Autodesk Inventor part; units mm, degrees
ref_plane "YZ Plane" through (0, 0, 0) normal (1, 0, 0) x (0, 1, 0)
ref_plane "XZ Plane" through (0, 0, 0) normal (0, 1, 0) x (-1, 0, 0)
ref_plane "XY Plane" through (0, 0, 0) normal (0, 0, 1) x (1, 0, 0)
sketch "Sketch1" plane through (0, 0, 0) normal (0, 1, 0) x (-1, 0, 0)
  line L0 (4.75, 4) -> (-4.75, 4)
  line L1 (-4.75, 4) -> (-4.75, -4)
  line L2 (-4.75, -4) -> (4.75, -4)
  line L3 (4.75, -4) -> (4.75, 4)
  line L4 (4.75, 4) -> (-4.75, -4) construction
  line L5 (-4.75, 4) -> (4.75, -4) construction
  point P0 (0, 0)
  dimension "d0" = 9.5
  dimension "d1" = 8
extrude "Extrusion1" add sketch "Sketch1" along normal blind 8
sketch "Sketch2" plane through (0, 8, 0) normal (0, 1, 0) x (1, 0, 0)
  circle A0 centre (-0.45, 0) radius 2
  line L0 (-4.75, 4) -> (-4.75, -4)
  line L1 (4.75, 4) -> (-4.75, 4)
  point P0 (0, 0)
  dimension "d4" = 4
  dimension "d5" = 4.3
  dimension "d6" = 4
extrude "Extrusion2" add sketch "Sketch2" along normal blind 3.2
sketch "Sketch3" plane through (-0.45, 11.2, 0) normal (0, 1, 0) x (1, 0, 0)
  point P0 (0.45, 0)
  point P1 (0, 0)
hole "Hole1" at (-0.45, 11.2, 0) direction (0, -1, 0) diameter 2.5 depth 8
sketch "Sketch4" plane through (0, 0, 0) normal (0, -1, 0) x (1, 0, 0)
  line L0 (-3.65, -1) -> (-3.85, -1)
  line L1 (-3.85, -1) -> (-3.85, 1)
  line L2 (-3.85, 1) -> (-3.65, 1)
  line L3 (-3.65, 1) -> (-3.65, -1)
  line L4 (-3.65, -1) -> (-3.85, 1) construction
  line L5 (-3.85, -1) -> (-3.65, 1) construction
  line L6 (3.65, -1) -> (3.85, -1)
  line L7 (3.85, -1) -> (3.85, 1)
  line L8 (3.85, 1) -> (3.65, 1)
  line L9 (3.65, 1) -> (3.65, -1)
  line L10 (3.65, -1) -> (3.85, 1) construction
  line L11 (3.85, -1) -> (3.65, 1) construction
  line L12 (4.75, 4) -> (4.75, -4)
  line L13 (-4.75, 4) -> (4.75, 4)
  point P0 (0, 0)
  point P1 (-3.75, 0)
  point P2 (3.75, 0)
  point P3 (3.65, 0)
  dimension "d16" = 0.2
  dimension "d17" = 2
  dimension "d18" = 0.2
  dimension "d19" = 2
  dimension "d20" = 7.5
  dimension "d21" = 1
  dimension "d22" = 4
extrude "Extrusion3" add sketch "Sketch4" along normal blind 5
fillet "Fillet1" radius 1 4 edges at (3.75, -5, -1) (3.75, -5, 1) (-3.75, -5, 1) (-3.75, -5, -1)
sketch "Sketch5" plane through (3.85, 0, 1) normal (1, 0, 0) x (0, 0, -1)
  line L0 (1, -2) -> (1, -4) construction
  line L1 (1.5, -2) -> (1.5, -4)
  line L2 (0.5, -4) -> (0.5, -2)
  arc A0 (1.5, -2) -> (0.5, -2) centre (1, -2) ccw
  arc A1 (0.5, -4) -> (1.5, -4) centre (1, -4) ccw
  line L3 (0, 0) -> (0, -4)
  arc A2 (0, -4) -> (2, -4) centre (1, -4) ccw
  point P0 (1, 0)
  point P1 (1, -3)
  dimension "d26" = 1
  dimension "d27" = 1
  dimension "d28" = 0.5
  dimension "d29" = 0.5
extrude "Extrusion4" cut sketch "Sketch5" against normal through all
sketch "Sketch6" plane through (-4.75, 0, -4) normal (-1, 0, 0) x (0, 0, 1)
  line L0 (3, 7.6) -> (5, 7.6)
  line L1 (5, 7.6) -> (5, 7.4)
  line L2 (5, 7.4) -> (3, 7.4)
  line L3 (3, 7.4) -> (3, 7.6)
  line L4 (3, 7.6) -> (5, 7.4) construction
  line L5 (5, 7.6) -> (3, 7.4) construction
  line L6 (0, 0) -> (0, 8)
  line L7 (0, 8) -> (8, 8)
  point P0 (4, 0)
  point P1 (4, 7.5)
  dimension "d32" = 2
  dimension "d33" = 0.2
  dimension "d34" = 4
  dimension "d35" = 0.5
extrude "Extrusion5" add sketch "Sketch6" along normal blind 5.7
fillet "Fillet2" radius 1 2 edges at (-10.45, 7.5, 1) (-10.45, 7.5, -1)
sketch "Sketch7" plane through (-4.75, 7.6, 1) normal (0, 1, 0) x (1, 0, 0)
  line L0 (-4.7, 1) -> (-3.7, 1) construction
  line L1 (-4.7, 0.5) -> (-3.7, 0.5)
  line L2 (-3.7, 1.5) -> (-4.7, 1.5)
  arc A0 (-4.7, 1.5) -> (-4.7, 0.5) centre (-4.7, 1) ccw
  arc A1 (-3.7, 0.5) -> (-3.7, 1.5) centre (-3.7, 1) ccw
  line L3 (0, 2) -> (-4.7, 2)
  arc A2 (-4.7, 2) -> (-4.7, 0) centre (-4.7, 1) ccw
  point P0 (4.75, 1)
  point P1 (-4.2, 1)
  dimension "d39" = 0.5
  dimension "d40" = 1
  dimension "d41" = 0.5
  dimension "d42" = 0.5
extrude "Extrusion6" cut sketch "Sketch7" against normal through all
properties part number "2.5mm jack"
Part model, mm, in its own coordinate system. A direction names the side the tool comes from. Round coordinates to 2 decimals unless told otherwise and drop trailing zeros. Write each loop counter-clockwise with the first axis right and the second up, starting at its lowest first coordinate (ties: lowest second). Pieces come first, ordered by that corner, then holes. Notation, with made-up numbers: (-34, -28) -> (25, -28) arc R22 ccw to (25, 8) -> close; hole circle Ø3 at (52.25, -12.75). An arc over 180 degrees is marked (long way). Return JSON: item names as keys, results as strings. Group by question number.
Q1. Which spindle directions (+Z, -Z, +X, -X, +Y, -Y) get a long thin tool onto all of the face, cutting with end or side? Do faces 1 (the flat face through (3.85, -1.9, -0.7)), 2 (the cylindrical face through (0.77, 7.14, -0.27)), 3 (the flat face through (3.65, -1.9, 0.7)). Say none if no direction does.
Q2. Saw through at D-D on z = 2.5. Write the cut outline in (x, y), plus the area to 3 significant figures.
Q3. Probe L1, parallel to X at y = 9.25, z = 0; L2, parallel to X at y = 5, z = 0; L3, parallel to Z at x = -0.45, y = 9. List the from-to ranges inside material, lowest first. Write a range as [from, to].
Q4. Saw through at A-A on x = -8.25. Write the cut outline in (y, z).
Q5. Pin check, flat tips, straight feed: pin 1 (2 mm diameter, centred on y = -2.5, z = -0.5, fed in from -X); pin 2 (4 mm diameter, centred on y = 2.5, z = 0.5, fed in from -X); pin 3 (0.6 mm diameter, centred on y = -3, z = 0, fed in from +X) (3 decimals). Stop position of each tip, or through.
Q6. Saw through at B-B on y = 5.75. Write the cut outline in (x, z).
Q7. Mould opens along X. For faces 4 (the flat face through (-3.85, -1.9, -0.7)), 5 (the cylindrical face through (-0.884, 9.578, -1.952)), 6 (the flat face through (0, 3.2, 0)) say: pulls with the +X half, pulls with the -X half, needs draft (parallel to the pull), parting line crosses it, or undercut.
Q8. Saw through at C-C on x = -0.45. Write the cut outline in (y, z).
Answer:
{
 "1": {"face 1": "+Z, -Z, +X, -Y", "face 2": "+Y", "face 3": "+Z, -Z, -Y"},
 "2": {"outline": "(-4.75, 0) -> (4.75, 0) -> (4.75, 8) -> (-4.75, 8) -> close", "area": "76.0 mm2"},
 "3": {"L1": "[-2.45, -1.7], [0.8, 1.55]", "L2": "[-4.75, -1.7], [0.8, 4.75]", "L3": "[-2, -1.25], [1.25, 2]"},
 "4": {"outline": "(7.4, -1) -> (7.6, -1) -> (7.6, -0.46) -> (7.4, -0.46) -> close; (7.4, 0.46) -> (7.6, 0.46) -> (7.6, 1) -> (7.4, 1) -> close"},
 "5": {"pin 1": "x = -3.85", "pin 2": "x = -4.75", "pin 3": "through"},
 "6": {"outline": "(-4.75, -4) -> (4.75, -4) -> (4.75, 4) -> (-4.75, 4) -> close; hole circle Ø2.5 at (-0.45, 0)"},
 "7": {"face 4": "pulls with the -X half", "face 5": "parting line crosses it", "face 6": "undercut"},
 "8": {"outline": "(0, -4) -> (8, -4) -> (8, -2) -> (11.2, -2) -> (11.2, -1.25) -> (3.2, -1.25) -> (3.2, 1.25) -> (11.2, 1.25) -> (11.2, 2) -> (8, 2) -> (8, 4) -> (0, 4) -> close"}
}
